Answer from the drawing. Dimensions are ordinates in mm from the lowest x, y and z of the part. Round coordinates to 2 decimals unless told otherwise and drop trailing zeros. Loops run counter-clockwise (first coordinate to the right, second up) from the corner with the lowest first, then second, coordinate; pieces in that order, holes last. Notation, with made-up numbers: (55, -13) -> (102, -13) arc R15 cw to (102, -1) -> close; hole circle Ø7 at (53.5, -10.75). An arc over 180 degrees is marked (long way). One line per question, with ' | ' between items.
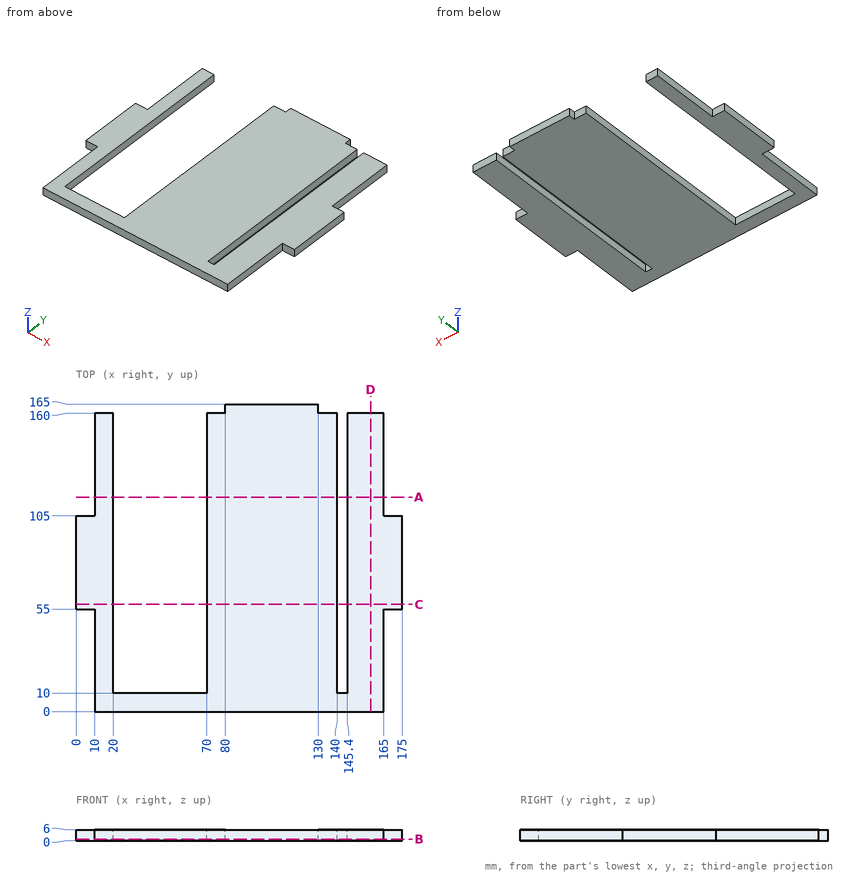
Q1. A cutting plane is placed at D-D on x = 158. Give the vertices of the cut face in (y, z).
Numbers:
outline: (0, 0) -> (160, 0) -> (160, 6) -> (0, 6) -> close
Q2. A cutting plane is placed at B-B on z = 0.9. Give the vertices of the cut face in (x, y).
Numbers:
outline: (0, 55) -> (10, 55) -> (10, 0) -> (165, 0) -> (165, 55) -> (175, 55) -> (175, 105) -> (165, 105) -> (165, 160) -> (145.4, 160) -> (145.4, 10) -> (140, 10) -> (140, 160) -> (130, 160) -> (130, 165) -> (80, 165) -> (80, 160) -> (70, 160) -> (70, 10) -> (20, 10) -> (20, 160) -> (10, 160) -> (10, 105) -> (0, 105) -> close
Q3. A cutting plane is placed at A-A on y = 115. Give the vertices of the cut face in (x, z), plus the area to 3 significant figures.
Numbers:
outline: (10, 0) -> (20, 0) -> (20, 6) -> (10, 6) -> close; (70, 0) -> (140, 0) -> (140, 6) -> (70, 6) -> close; (145.4, 0) -> (165, 0) -> (165, 6) -> (145.4, 6) -> close | area: 598 mm^2
Q4. Given pin 1 Ø3 at (y, z) = (119, 2) entering from -X; pin 2 Ø3 at (y, z) = (139, 2.5) entering from +X; pin 3 Ø1.8 at (x, z) = (4.5, 2) entering from +Y, each flat-ended and moving along its own axis, determine where each tip first touches the part or whether it passes through.
Numbers:
pin 1: x = 10 | pin 2: x = 165 | pin 3: y = 105
Q5. A cutting plane is placed at C-C on y = 57.5. Give the vertices of the cut face in (x, z), plus the area to 3 significant figures.
Numbers:
outline: (0, 0) -> (20, 0) -> (20, 6) -> (0, 6) -> close; (70, 0) -> (140, 0) -> (140, 6) -> (70, 6) -> close; (145.4, 0) -> (175, 0) -> (175, 6) -> (145.4, 6) -> close | area: 718 mm^2
Q6. Find the intervals of material crossed by line 1 (X direction, y = 16, z = 0.45); line 2 (X direction, y = 76, z = 4); line 3 (Y direction, x = 167.5, z = 2.35), in increasing order. Write a range as from..to.
Numbers:
line 1: 10..20, 70..140, 145.4..165 | line 2: 0..20, 70..140, 145.4..175 | line 3: 55..105
